from build123d import *

# Parameters (mm, degrees)
SKETCH2_W           = 15
SKETCH2_H           = 60
BOSS_EXTRUDE1_DEPTH = 12.5
SKETCH3_W           = 8
SKETCH3_H           = 12.5
CUT_EXTRUDE1_DEPTH  = 36.794552658
SKETCH4_R           = 2.25
CUT_EXTRUDE2_DEPTH  = 36.288099977
FILLET1_R           = 5
FILLET2_R           = 4
SKETCH5_R           = 6
CUT_EXTRUDE3_DEPTH  = 36.794552658
SKETCH6_R           = 10
CUT_EXTRUDE4_DEPTH  = 10


with BuildPart() as part:
    # Sketch2 → Boss-Extrude1 (new, symmetric)
    with BuildSketch(Plane.XY):
        Rectangle(SKETCH2_W, SKETCH2_H)
    extrude(amount=BOSS_EXTRUDE1_DEPTH, both=True)

    # Sketch3 → Cut-Extrude1 (cut, through all)
    with BuildSketch(Plane(origin=(7.5, 0, 0), x_dir=(0, 0, -1), z_dir=(1, 0, 0))):
        with Locations((-8.5, -23.75)):
            Rectangle(SKETCH3_W, SKETCH3_H)
        with Locations((8.5, -23.75)):
            Rectangle(SKETCH3_W, SKETCH3_H)
        with Locations((8.5, 23.75)):
            Rectangle(SKETCH3_W, SKETCH3_H)
        with Locations((-8.5, 23.75)):
            Rectangle(SKETCH3_W, SKETCH3_H)
    extrude(amount=-CUT_EXTRUDE1_DEPTH, mode=Mode.SUBTRACT)

    # Sketch4 → Cut-Extrude2 (cut, through all)
    with BuildSketch(Plane.XY.offset(4.5)):
        with Locations((-2.5, 25)):
            Circle(SKETCH4_R)
        with Locations((-2.5, -24.5)):
            Circle(SKETCH4_R)
    extrude(amount=-CUT_EXTRUDE2_DEPTH, mode=Mode.SUBTRACT)

    # Fillet1
    fillet1_edges = [part.edges().sort_by_distance(p)[0] for p in [
        (0, 17.5, 12.5),
        (0, 17.5, -12.5),
        (0, -17.5, -12.5),
        (0, -17.5, 12.5),
    ]]
    fillet(fillet1_edges, radius=FILLET1_R)

    # Fillet2
    fillet2_edges = [part.edges().sort_by_distance(p)[0] for p in [
        (7.5, -30, 0),
        (-7.5, -30, 0),
        (-7.5, 30, 0),
        (7.5, 30, 0),
    ]]
    fillet(fillet2_edges, radius=FILLET2_R)

    # Sketch5 → Cut-Extrude3 (cut, through all)
    with BuildSketch(Plane.ZY.offset(7.5)):
        with Locations(Location((0, 0, 0), (0, 0, 270))):
            Circle(SKETCH5_R)
    extrude(amount=-CUT_EXTRUDE3_DEPTH, mode=Mode.SUBTRACT)

    # Sketch6 → Cut-Extrude4 (cut)
    with BuildSketch(Plane.ZY.offset(7.5)):
        with Locations(Location((0, 0, 0), (0, 0, 270))):
            Circle(SKETCH6_R)
    extrude(amount=-CUT_EXTRUDE4_DEPTH, mode=Mode.SUBTRACT)


solid = part.part
Part model, mm, in its own coordinate system. A direction names the side the tool comes from. Give positions to 0.01 mm unless a question says otherwise; leave off trailing zeros. Loops run counter-clockwise (first coordinate to the right, second up) from the corner with the lowest first, then second, coordinate; pieces in that order, holes last. Notation, with made-up numbers: M -2,64 L 9,64 A34 ccw 9,101 Z; hole C 72,-2 d9. An arc over 180 degrees is marked long. Put each result on its own line as item: value. Start each with the question number.
1) 3-axis set-ups, long thin cutter, end or side, ignore diameter. For faces 4 (the flat face through (0, -24, 4.5)), 5 (the cylindrical face through (-0.11, 16, 11.07)), 6 (the flat face through (0, 24, -4.5)), 7 (the flat face through (2.5, 0, -7)): which of +Z, -Z, +X, -X, +Y, -Y reach the whole face in a straight line?
2) Saw through at A-A (z = 0). List the corners of the cut face in (x, y), then the cut area to 3 significant figures.
3) Saw through at D-D (y = 8). List the corners of the cut face in (x, z), then the cut area to 3 significant figures.
4) Saw through at C-C (x = -2.5). List the corners of the cut face in (y, z), then the cut area to 3 significant figures.
5) Saw through at B-B (y = 25). List the corners of the cut face in (x, z).
6) Probe probe 1 along Z at (x, y) = (4.7, 0); probe 2 along Z at (x, y) = (-0.25, 0); probe 3 along Y at (x, z) = (-3.5, 2). List the from-to ranges inside material, lowest first.
7) Flat gauge pins, fed straight in: pin 1 (2.5 mm diameter, centred on x = -0.5, z = 5.5, fed in from +Y); pin 2 (3 mm diameter, centred on x = 4, y = -16, fed in from -Z); pin 3 (10 mm diameter, centred on y = -2.5, z = -3, fed in from -X); pin 4 (4 mm diameter, centred on x = -2, y = 26.5, fed in from -Z). Where does each tip first touch, or does it go through?
8) Pull direction Y, two halves, no side cores. Call faces 1 (the flat face through (0, 17.5, 6)), 2 (the cylindrical face through (4.965, -5.723, 1.802)), 3 (the flat face through (0, -17.5, -6)): +Y half, -Y half, draft (parallel to the pull), parting line (faces both ways), or undercut.
Numbers:
1. face 4: +Z, +X, -X, -Y
1. face 5: +Z, +X, -X, +Y
1. face 6: -Z, +X, -X, +Y
1. face 7: -X
2. outline: M -7.5,-26 A4 ccw -3.5,-30 L 3.5,-30 A4 ccw 7.5,-26 L 7.5,-6 L 2.5,-6 L 2.5,-10 L -7.5,-10 Z; M -7.5,10 L 2.5,10 L 2.5,6 L 7.5,6 L 7.5,26 A4 ccw 3.5,30 L -3.5,30 A4 ccw -7.5,26 Z; hole C -2.5,-24.5 d4.5; hole C -2.5,25 d4.5
2. area: 594 mm^2
3. outline: M -7.5,-12.5 L 7.5,-12.5 L 7.5,12.5 L -7.5,12.5 L -7.5,6 L 2.5,6 L 2.5,-6 L -7.5,-6 Z
3. area: 255 mm^2
4. outline: M -30,-4.5 L -26.75,-4.5 L -26.75,4.5 L -30,4.5 Z; M -22.25,-4.5 L -17.5,-4.5 L -17.5,-7.5 A5 ccw -12.5,-12.5 L 12.5,-12.5 A5 ccw 17.5,-7.5 L 17.5,-4.5 L 22.75,-4.5 L 22.75,4.5 L 17.5,4.5 L 17.5,7.5 A5 ccw 12.5,12.5 L -12.5,12.5 A5 ccw -17.5,7.5 L -17.5,4.5 L -22.25,4.5 Z; M 27.25,-4.5 L 30,-4.5 L 30,4.5 L 27.25,4.5 Z; hole C 0,0 d20
4. area: 683 mm^2
5. outline: M -7.5,-4.5 L -4.75,-4.5 L -4.75,4.5 L -7.5,4.5 Z; M -0.25,-4.5 L 7.5,-4.5 L 7.5,4.5 L -0.25,4.5 Z
6. probe 1: -12.5 to -6, 6 to 12.5
6. probe 2: -12.5 to -10, 10 to 12.5
6. probe 3: -30 to -26.52, -22.48 to -9.8, 9.8 to 22.98, 27.02 to 30
7. pin 1: y = 30
7. pin 2: z = -12.08
7. pin 3: x = 2.5
7. pin 4: z = -4.5
8. face 1: +Y half
8. face 2: undercut
8. face 3: -Y half
